```python
from build123d import *

# Parameters (mm, degrees)
F0_W     = 300
F0_H     = 300
F1_DEPTH = 10
F2_R     = 10
F2_R_2   = 5
F2_R_3   = 9.83343
F3_DEPTH = 25
F4_R     = 5
F5_DEPTH = 13.4


with BuildPart() as f1:
    # F0 (on Top) → F1 (new body)
    with BuildSketch(Plane.XY):
        with Locations((-93.317212, 97.135217)):
            Rectangle(F0_W, F0_H)
    extrude(amount=F1_DEPTH)

    # F2 (on Front) → F3 (join)
    with BuildSketch(Plane.XZ):
        with Locations((-251.922578, 5.191812)):
            Circle(F2_R)
        with Locations((-251.922578, 5.191812)):
            Circle(F2_R_2, mode=Mode.SUBTRACT)
        with Locations((64.999998, 5)):
            Circle(F2_R_3)
    extrude(amount=F3_DEPTH)

    # F4 (on face) → F5 (cut)
    with BuildSketch(Plane.XZ.offset(25)):
        with BuildLine():
            Line((56.682788, 10), (56.682788, 0))
            Line((56.682788, 0), (56.532628, 0))
            ThreePointArc((56.532628, 0), (74.833428, 5.000001), (56.532628, 10))
            Line((56.532628, 10), (56.682788, 10))
        make_face()
        with Locations((64.999998, 5)):
            Circle(F4_R, mode=Mode.SUBTRACT)
    extrude(amount=-F5_DEPTH, mode=Mode.SUBTRACT)


solid = f1.part
```
Verification items for the finished model (mm, model axes). A direction names the side the tool comes from. Round coordinates to 2 decimals unless told otherwise and drop trailing zeros. Write each loop counter-clockwise with the first axis right and the second up, starting at its lowest first coordinate (ties: lowest second). Pieces come first, ordered by that corner, then holes.
1. Access from +Z, -Z, +X, -X, +Y, -Y to the whole of each face (thin tool, end or side, straight path). Record for faces 4 (the flat face through (-95, 247.135, 5)), 5 (the flat face through (65, -25, 5)), 6 (the flat face through (56.683, 122, 5)), 7 (the cylindrical face through (69.619, -18.394, 3.085)), 8 (the cylindrical face through (-261.91, -12.32, 5.72)).
2. Section check A-A on y = 53. Enter the section's corners in (x, z), plus the area to 3 significant figures.
3. Section check B-B on x = -98.5. Enter the section's corners in (y, z).
4. Draft check along X on faces 1 (the flat face through (56.683, -33, 5)), 2 (the flat face through (-243.317, 95, 5)), 3 (the flat face through (66, 0, 5)). Enter one of: +X half, -X half, draft (parallel to the pull), parting line (faces both ways), or undercut.
5. Scan lines: L1, parallel to Z at x = 5, y = -10.5; L2, parallel to X at y = 97.5, z = 1; L3, parallel to Y at x = 58, z = 3.75. Record each from-to range of solid material in increasing order.
6. Gauge pin test, flat ends, axial feed: P1, Ø5, axis at y = 146, z = 5.5, coming from the +X side; P2, Ø8, axis at x = 66.5, z = 4.5, coming from the -Y side; P3, Ø12, axis at x = -29, y = 114.5, coming from the -Z side. Record the tip position at first contact, or that the pin passes through.
Answer:
1. face 4: +Z, -Z, +X, -X, +Y
1. face 5: +Z, -Z, +X, -Y
1. face 6: +Z, -Z, +X, +Y
1. face 7: -Y
1. face 8: +Y, -Y
2. outline: (-243.32, 0) - (56.68, 0) - (56.68, 10) - (-243.32, 10) - close
2. area: 3,000 mm2
3. outline: (-52.86, 0) - (247.14, 0) - (247.14, 10) - (-52.86, 10) - close
4. face 1: undercut
4. face 2: -X half
4. face 3: draft
5. L1: z = 0 to 10
5. L2: x = -243.32 to 56.68
5. L3: y = -11.6 to 0
6. P1: stops at x = 56.68
6. P2: stops at y = -25
6. P3: stops at z = 0
